Check sheet for the modelled part. Datum: model origin and axes. Units: mm. A direction names the side the tool comes from. Give positions to 0.01 mm unless a question says otherwise; leave off trailing zeros. Order: outer loops, then holes, each group sorted by start corner. A loop starts at its lowest first (then second) coordinate and runs counter-clockwise, first axis right, second up. Notation, with made-up numbers: (25.5, 50) -> (79.5, 50) arc R15 ccw to (79.5, 69) -> close; hole circle Ø3 at (81, 77). An arc over 180 degrees is marked (long way). Answer in a Markdown table with one row per item. Add a question column.
(1) Set-up check for faces 1 (the face through (2, 5, 61)), 2 (the face through (27, -20, -15)), 3 (the face through (71.728, -10.14, -43.722)): record each of +Z, -Z, +X, -X, +Y, -Y from which the full face is reachable in a straight line by a thin tool's end or side.
(2) Go/stop test with flat-tipped pins: pin 1 (12 mm diameter, centred on y = -12.5, z = 105, fed in from -X); pin 2 (10 mm diameter, centred on y = -10, z = 75, fed in from -X); pin 3 (12 mm diameter, centred on x = -34.5, z = 103.5, fed in from -Y). Record where each tip stops, or that it passes through.
(3) Cross-section at C-C (z = -75.5). Record the cut outline in (x, y), then the cut area to 3 significant figures.
(4) Cross-section at A-A (y = -12). Record the cut outline in (x, z), then the cut area to 3 significant figures.
(5) Release check for a two-part mould opening along X. For faces 4 (the face through (70.366, -10.14, 42.935)), 5 (the face through (-6, 19, 6)), 6 (the face through (8.86, 13.42, 28.14)) record: released by +X, released by -X, zero draft, split by the parting line, or undercut.
(6) Cross-section at B-B (x = 106.5). Record the cut outline in (y, z).
(7) Cross-section at D-D (x = -98.5). Record the cut outline in (y, z).
(8) Thickness scan on L1, parallel to X at y = 18.45, z = 0; L2, parallel to X at y = -2.5, z = 112; L3, parallel to Z at x = 62.5, y = -3 (3 decimals). Record the ranges inside material, lowest first. Write a range as [from, to].
```python
from build123d import *
from build123d.topology import SkipClean

# Parameters (mm, degrees)
SKETCH_1_R               = 141.4
EXTRUDE_1_DEPTH          = 5
SKETCH_2_R               = 50
EXTRUDE_2_DEPTH          = 3
SKETCH_3_R               = 29.5
EXTRUDE_3_DEPTH          = 11
SKETCH_4_R               = 27
CUT_EXTRUDE_1_DEPTH      = 16
SKETCH_5_R               = 3
SKETCH_5_R_2             = 1.5
CUT_EXTRUDE_2_DEPTH      = 201.608873184
EXTRUDE_START            = 20
EXTRUDE_1_2_DEPTH        = 20
PATTERN_CIRCULAR_1_COUNT = 6


with BuildPart() as part:
    # 草图1 → Extrude 1 (new body)
    with BuildSketch(Plane(origin=(0, 0, 0), x_dir=(1, 0, 0), z_dir=(0, 1, 0))):
        with Locations(Location((0, 0, 0), (0, 0, 270))):
            Circle(SKETCH_1_R)
    extrude(amount=EXTRUDE_1_DEPTH)

    # 草图2 → 凸台-拉伸2 (add)
    with BuildSketch(Plane(origin=(0, 5, 0), x_dir=(1, 0, 0), z_dir=(0, 1, 0))):
        with Locations(Location((0, 0, 0), (0, 0, 270))):
            Circle(SKETCH_2_R)
    extrude(amount=EXTRUDE_2_DEPTH)

    # 草图3 → 凸台-拉伸3 (add)
    with BuildSketch(Plane(origin=(0, 8, 0), x_dir=(1, 0, 0), z_dir=(0, 1, 0))):
        with Locations(Location((0, 0, 0), (0, 0, 270))):
            Circle(SKETCH_3_R)
    extrude(amount=EXTRUDE_3_DEPTH)

    # 草图4 → 切除-拉伸1 (cut)
    with BuildSketch(Plane.XZ):
        with Locations(Location((0, 0, 0), (0, 0, 270))):
            Circle(SKETCH_4_R)
    extrude(amount=-CUT_EXTRUDE_1_DEPTH, mode=Mode.SUBTRACT)

    # 草图5 → 切除-拉伸2 (cut, through all)
    with BuildSketch(Plane.XZ.offset(-16)):
        with Locations(Location((0, 0, 0), (0, 0, 270))):
            Circle(SKETCH_5_R)
        with Locations(Location((0, 7, 0), (0, 0, 270))):
            Circle(SKETCH_5_R_2)
        with Locations(Location((7, 0, 0), (0, 0, 270))):
            Circle(SKETCH_5_R_2)
        with Locations(Location((0, -7, 0), (0, 0, 270))):
            Circle(SKETCH_5_R_2)
        with Locations(Location((-7, 0, 0), (0, 0, 270))):
            Circle(SKETCH_5_R_2)
    extrude(amount=-CUT_EXTRUDE_2_DEPTH, mode=Mode.SUBTRACT)

    # 草图6 → Extrude 1 2 (add)
    with SkipClean():  # the faces are left unmerged after this step: merging them gives an invalid solid
        with BuildSketch(Plane.XZ.offset(EXTRUDE_START)):
            with BuildLine():
                Line((-23.382685902, 13.5), (-122.455992095, 70.7))
                ThreePointArc((-122.455992095, 70.7), (-70.7, 122.455992095), (0, 141.4))
                Line((0, 141.4), (0, 27))
                Line((0, 27), (-2, 27))
                Line((-2, 27), (-2, 139.385652059))
                ThreePointArc((-2, 139.385652059), (-69.7, 120.723941288), (-119.711515606, 71.424876837))
                Line((-119.711515606, 71.424876837), (-22.382685902, 15.232050808))
                Line((-22.382685902, 15.232050808), (-23.382685902, 13.5))
            make_face()
        extrude_1_2 = extrude(amount=-EXTRUDE_1_2_DEPTH)

    # 阵列(圆周)1: Extrude 1 2 ×6 about axis
    pattern_circular_1_axis = Axis((0, 0, 0), (0, 1, 0))
    for i in range(1, PATTERN_CIRCULAR_1_COUNT):
        add(extrude_1_2.rotate(pattern_circular_1_axis, i * 360 / PATTERN_CIRCULAR_1_COUNT))


solid = part.part
```
Answer below:
| question | item | result |
|---|---|---|
| 1 | face 1 | +Y |
| 1 | face 2 | +Z, -Z, +X, -X, -Y |
| 1 | face 3 | -Y |
| 2 | pin 1 | stops at x = -100.96 |
| 2 | pin 2 | stops at x = -122.86 |
| 2 | pin 3 | stops at y = 0 |
| 3 | outline | (-119.56, -20) -> (-117.18, -20) -> (-117.18, 0) -> (-2, 0) -> (-2, -20) -> (2, -20) -> (2, 0) -> (117.18, 0) -> (117.18, -20) -> (119.56, -20) -> (119.56, 5) -> (-119.56, 5) -> close |
| 3 | area | 1,370 mm² |
| 4 | outline | circle Ø282.8 at (0, 0); hole (-121.71, -67.96) -> (-24.38, -11.77) -> (-22.38, -15.23) -> (-119.71, -71.42) arc R139.4 ccw to (-2, -139.39) -> (-2, -27) -> (2, -27) -> (2, -139.39) arc R139.4 ccw to (119.71, -71.42) -> (22.38, -15.23) -> (24.38, -11.77) -> (121.71, -67.96) arc R139.4 ccw to (121.71, 67.96) -> (24.38, 11.77) -> (22.38, 15.23) -> (119.71, 71.42) arc R139.4 ccw to (2, 139.39) -> (2, 27) -> (-2, 27) -> (-2, 139.39) arc R139.4 ccw to (-119.71, 71.42) -> (-22.38, 15.23) -> (-24.38, 11.77) -> (-121.71, 67.96) arc R139.4 ccw to start |
| 4 | area | 4,460 mm² |
| 5 | face 4 | undercut |
| 5 | face 5 | zero draft |
| 5 | face 6 | split by the parting line |
| 6 | outline | (-20, -93.01) -> (5, -93.01) -> (5, 93.01) -> (-20, 93.01) -> (-20, 89.95) -> (0, 89.95) -> (0, 63.8) -> (-20, 63.8) -> (-20, 59.18) -> (0, 59.18) -> (0, -59.18) -> (-20, -59.18) -> (-20, -63.8) -> (0, -63.8) -> (0, -89.95) -> (-20, -89.95) -> close |
| 7 | outline | (-20, -101.45) -> (5, -101.45) -> (5, 101.45) -> (-20, 101.45) -> (-20, 98.64) -> (0, 98.64) -> (0, 59.18) -> (-20, 59.18) -> (-20, 54.56) -> (0, 54.56) -> (0, -54.56) -> (-20, -54.56) -> (-20, -59.18) -> (0, -59.18) -> (0, -98.64) -> (-20, -98.64) -> close |
| 8 | L1 | x = [-29.5, -8.5], [-5.5, -3], [3, 5.5], [8.5, 29.5] |
| 8 | L2 | x = [-86.31, -83], [-2, 2], [83, 86.31] |
| 8 | L3 | z = [-126.837, -124.604], [-38.394, -33.775], [33.775, 38.394], [124.604, 126.837] |
